from build123d import *

# Parameters (mm, degrees)
F1_DEPTH = 20
F0_R     = 2
F2_DEPTH = 3
F3_DEPTH = 4
F5_DEPTH = 3.25
F6_R     = 2
F7_DEPTH = 29.5010001


# Not quite as in the source:
# - a feature names something its author has since deleted; it is built from what else it names


with BuildPart() as f1:
    # F0 (on Top) → F1 (new body)
    with BuildSketch(Plane.XY):
        with BuildLine():
            ThreePointArc((-18.2551362635, 3.1646558729), (18.5, 0.1646558729), (-18.2551362635, -2.8353441271))
            Line((-18.2551362635, -2.8353441271), (-21.289668856, -2.8353441271))
            Line((-21.289668856, -2.8353441271), (-33.5, -2.8353441271))
            Line((-33.5, -2.8353441271), (-33.5, -5.8353441271))
            Line((-33.5, -5.8353441271), (-33.5, -7.8353441271))
            Line((-33.5, -7.8353441271), (-20.4217309456, -7.8353441271))
            ThreePointArc((-20.4217309456, -7.8353441271), (8.7176252261, -19.2755005117), (18.3885107603, 10.4978639134))
            ThreePointArc((18.3885107603, 10.4978639134), (-0.3478610365, 21.6643338769), (-19.2053350681, 10.7036152553))
            ThreePointArc((-19.2053350681, 10.7036152553), (-19.8551354356, 9.4540669672), (-20.4217309456, 8.1646558729))
            Line((-20.4217309456, 8.1646558729), (-33.5, 8.1646558729))
            Line((-33.5, 8.1646558729), (-33.5, 6.1646558729))
            Line((-33.5, 6.1646558729), (-33.5, 3.1646558729))
            Line((-33.5, 3.1646558729), (-21.289668856, 3.1646558729))
            Line((-21.289668856, 3.1646558729), (-18.2551362635, 3.1646558729))
        make_face()
    extrude(amount=F1_DEPTH)

    # F0 (on Top) → F2 (join)
    with BuildSketch(Plane.XY):
        with BuildLine():
            ThreePointArc((-19.2053350681, 10.7036152553), (-0.3478610365, 21.6643338769), (18.3885107603, 10.4978639134))
            ThreePointArc((18.3885107603, 10.4978639134), (14.2120337074, 27.5685018888), (19.1172770705, 44.4441716239))
            ThreePointArc((19.1172770705, 44.4441716239), (13.4958098431, 42.2172179553), (9.8397882001, 47.0332040616))
            Line((9.8397882001, 47.0332040616), (-10.1602117999, 47.0332040616))
            ThreePointArc((-10.1602117999, 47.0332040616), (-13.8544265436, 42.2067224379), (-19.4781817457, 44.512264644))
            ThreePointArc((-19.4781817457, 44.512264644), (-14.8414845345, 27.6442586076), (-19.2053350681, 10.7036152553))
        make_face()
        with BuildLine():
            add(Edge.make_bspline(
                [(7.5, 31.9373905659), (7.5, 37.9995683924), (-3.75, 34.9684794791), (-15, 31.9373905659), (-3.75, 28.9063016526), (7.5, 25.8752127394), (7.5, 31.9373905659)],
                knots=[0, 0, 0, 2.0943951024, 2.0943951024, 4.1887902048, 4.1887902048, 6.2831853072, 6.2831853072, 6.2831853072], degree=2, weights=[1, 0.5, 1, 0.5, 1, 0.5, 1]))
        make_face(mode=Mode.SUBTRACT)
        with BuildLine():
            ThreePointArc((-10.1602117999, 47.0332040616), (-16.4659970562, 51.8596856854), (-19.4781817457, 44.512264644))
            ThreePointArc((-19.4781817457, 44.512264644), (-13.8544265436, 42.2067224379), (-10.1602117999, 47.0332040616))
        make_face()
        with Locations((-15.1602117999, 47.0332040616)):
            Circle(F0_R, mode=Mode.SUBTRACT)
        with BuildLine():
            ThreePointArc((9.8397882001, 47.0332040616), (13.4958098431, 42.2172179553), (19.1172770705, 44.4441716239))
            ThreePointArc((19.1172770705, 44.4441716239), (19.6557743064, 45.6892257046), (19.8397882001, 47.0332040616))
            ThreePointArc((19.8397882001, 47.0332040616), (14.8397882001, 52.0332040616), (9.8397882001, 47.0332040616))
        make_face()
        with BuildLine():
            ThreePointArc((16.8397882001, 47.0332040616), (14.8397882001, 45.0332040616), (12.8397882001, 47.0332040616))
            ThreePointArc((12.8397882001, 47.0332040616), (14.8397882001, 49.0332040616), (16.8397882001, 47.0332040616))
        make_face(mode=Mode.SUBTRACT)
    extrude(amount=F2_DEPTH)

    # F0 (on Top) → F3 (join)
    with BuildSketch(Plane.XY):
        with BuildLine():
            ThreePointArc((-10.1602117999, 47.0332040616), (-16.4659970562, 51.8596856854), (-19.4781817457, 44.512264644))
            ThreePointArc((-19.4781817457, 44.512264644), (-13.8544265436, 42.2067224379), (-10.1602117999, 47.0332040616))
        make_face()
        with Locations((-15.1602117999, 47.0332040616)):
            Circle(F0_R, mode=Mode.SUBTRACT)
        with BuildLine():
            ThreePointArc((9.8397882001, 47.0332040616), (13.4958098431, 42.2172179553), (19.1172770705, 44.4441716239))
            ThreePointArc((19.1172770705, 44.4441716239), (19.6557743064, 45.6892257046), (19.8397882001, 47.0332040616))
            ThreePointArc((19.8397882001, 47.0332040616), (14.8397882001, 52.0332040616), (9.8397882001, 47.0332040616))
        make_face()
        with BuildLine():
            ThreePointArc((16.8397882001, 47.0332040616), (14.8397882001, 45.0332040616), (12.8397882001, 47.0332040616))
            ThreePointArc((12.8397882001, 47.0332040616), (14.8397882001, 49.0332040616), (16.8397882001, 47.0332040616))
        make_face(mode=Mode.SUBTRACT)
    extrude(amount=F3_DEPTH)

    # F4 (on face) → F5 (cut)
    with BuildSketch(Plane.XZ.offset(7.8353441271)):
        Polygon((-31.0858654728, 12.3815698604), (-31.0858654728, 7.6184301396), (-26.9608654728, 5.2368602792), (-22.8358654728, 7.6184301396), (-22.8358654728, 12.3815698604), (-26.9608654728, 14.7631397208), align=None)
    extrude(amount=-F5_DEPTH, mode=Mode.SUBTRACT)

    # F6 (on face) → F7 (cut, through all)
    with BuildSketch(Plane(origin=(0, 8.1646558729, 0), x_dir=(-1, 0, 0), z_dir=(0, 1, 0))):
        with Locations((26.9608654728, 10)):
            Circle(F6_R)
    extrude(amount=-F7_DEPTH, mode=Mode.SUBTRACT)


solid = f1.part
Design review of the part built by this model. Coordinates are the model's own, in mm. A direction names the side the tool comes from. Give positions to 0.01 mm unless a question says otherwise; leave off trailing zeros. Loops run counter-clockwise (first coordinate to the right, second up) from the corner with the lowest first, then second, coordinate; pieces in that order, holes last. Notation, with made-up numbers: (68.5, 75) -> (112.5, 75) arc R18 ccw to (112.5, 96) -> close; hole circle Ø5 at (62, 16). An arc over 180 degrees is marked (long way). One line per question, with ' | ' between items. Start each with the question number.
(1) We need section B-B (y = -13). State the section outline as (x, z) points.
(2) We need section C-C (x = -12). State the section outline as (y, z) points, and give its area (3 significant figures).
(3) We need section A-A (z = 10). State the section outline as (x, y) points, and give its area (3 significant figures).
(4) Insertion check: P1, Ø12, axis at x = -11, y = 11.5, coming from the -Z side; P2, Ø1, axis at x = 3.5, z = 9.5, coming from the -Y side; P3, Ø4, axis at x = -28, z = 10, coming from the -Y side; P4, Ø10.5, axis at x = -25.5, z = 7.5, coming from the -Y side. Each pin has a flat end and moves straight along its axis. Give the tip position at first contact, or say it passes through.
(5) We need section D-D (z = 18.75). State the section outline as (x, y) points.
(6) Draft analysis for pull direction Y (two halves, no side actions). For faces 4 (the face through (-24, 3.165, 10)), 5 (the face through (16.85, 51.61, 2.42)), 6 (the face through (-29, -4.585, 9)), 7 (the face through (-24.963, 5.7, 10.088)), state which applies: +Y half, -Y half, draft (parallel to the pull), parting line (faces both ways), or undercut.
(7) For faces 1 (the face through (0, 47.033, 1)), 2 (the face through (-24.93, -6.23, 6.41)), 3 (the face through (-15.23, 44.88, 4)), list the 3-axis set-ups (+Z, -Z, +X, -X, +Y, -Y) from which the entire face can be reached by the end or side of a thin tool; tool diameter is ignored.
(8) For line 1 (X direction, y = 47, z = 1); line 2 (Y direction, x = -26, z = 5); line 3 (Y direction, x = -28.5, z = 8.5), list the stretches that pass through material, from the lowest coordinate up.
The answers:
1) outline: (-17.46, 0) -> (-13, 0) -> (-13, 20) -> (-17.46, 20) -> close; (13, 0) -> (16.53, 0) -> (16.53, 20) -> (13, 20) -> close
2) outline: (-17.98, 0) -> (-13.92, 0) -> (-13.92, 20) -> (-17.98, 20) -> close; (14.24, 0) -> (50.91, 0) -> (50.91, 4) -> (43.16, 4) -> (43.16, 3) -> (18.31, 3) -> (18.31, 20) -> (14.24, 20) -> close | area: 268 mm^2
3) outline: (-33.5, -7.84) -> (-31.09, -7.84) -> (-31.09, -4.59) -> (-28.96, -4.59) -> (-28.96, -2.84) -> (-33.5, -2.84) -> close; (-33.5, 3.16) -> (-28.96, 3.16) -> (-28.96, 8.16) -> (-33.5, 8.16) -> close; (-24.96, -4.59) -> (-22.84, -4.59) -> (-22.84, -7.84) -> (-20.42, -7.84) arc R21.5 ccw (long way) to (-20.42, 8.16) -> (-24.96, 8.16) -> (-24.96, 3.16) -> (-18.26, 3.16) arc R18.5 cw (long way) to (-18.26, -2.84) -> (-24.96, -2.84) -> close | area: 425 mm^2
4) P1: stops at z = 0 | P2: stops at y = -21.05 | P3: stops at y = -4.59 | P4: stops at y = -8.25
5) outline: (-33.5, -7.84) -> (-20.42, -7.84) arc R21.5 ccw (long way) to (-20.42, 8.16) -> (-33.5, 8.16) -> (-33.5, 3.16) -> (-18.26, 3.16) arc R18.5 cw (long way) to (-18.26, -2.84) -> (-33.5, -2.84) -> close
6) face 4: undercut | face 5: undercut | face 6: -Y half | face 7: draft
7) face 1: +Z, -Z, +Y | face 2: -Y | face 3: +Z, +X, -X, +Y
8) line 1: x = -20.16 to -17.16, -13.16 to 12.84, 16.84 to 19.84 | line 2: y = -7.84 to -2.84, 3.16 to 8.16 | line 3: y = -4.59 to -2.84, 3.16 to 8.16
